from build123d import *

# Parameters (mm, degrees)
F0_R     = 4.5
F0_R_2   = 2.95
F1_DEPTH = 10
F0_R_3   = 15.5
F2_DEPTH = 10
F3_DEPTH = 15


with BuildPart() as f1:
    # F0 (on Top) → F1 (new body)
    with BuildSketch(Plane.XY):
        Circle(F0_R)
        Circle(F0_R_2, mode=Mode.SUBTRACT)
    extrude(amount=F1_DEPTH)

    # F0 (on Top) → F2 (join)
    with BuildSketch(Plane.XY):
        Circle(F0_R_3)
        Circle(F0_R, mode=Mode.SUBTRACT)
    extrude(amount=-F2_DEPTH)

    # F3 (add): a face of the model
    f3_faces = [f1.faces().sort_by_distance(p)[0] for p in [
        (-4.3727207794, 0, 0),
    ]]
    extrude(f3_faces, amount=F3_DEPTH)


solid = f1.part
The listing builds one solid part. Answer for the finished solid, in the listing's coordinates (mm). A direction names the side the tool comes from. Coordinates: 2 decimals unless noted, no trailing zeros. Order: outer loops, then holes, each group sorted by start corner. A loop starts at its lowest first (then second) coordinate and runs counter-clockwise, first axis right, second up. Notation, with made-up numbers: (82.5, 77.5) -> (98.5, 77.5) arc R21 cw to (98.5, 99.5) -> close; hole circle Ø9 at (21, 73). An arc over 180 degrees is marked (long way). Answer in a Markdown table with one row per item. Add a question column.
Item 1: Find section D-D (x = 8). Write down the section's boundary in (y, z), then the cut area to 3 significant figures.
Item 2: Which of the six approach directions +Z, -Z, +X, -X, +Y, -Y give full straight-line access (tool end or side, diameter ignored) to faces 1 (the face through (1, -3, -15)), 2 (the face through (-4, -3, -10)), 3 (the face through (-0.59, 4.46, 4.93))?
Item 3: Find section C-C (z = -1.5). Write down the section's boundary in (x, y), then the cut area to 3 significant figures.
Item 4: Each of these flat-tipped pins is pushed along its axis until it touches: P1, Ø10, axis at x = 10, y = -5, coming from the -Z side; P2, Ø5.5, axis at x = 0, y = 0, coming from the +Z side; P3, Ø5, axis at y = -4.5, z = -1, coming from the +X side; P4, Ø10, axis at y = 11, z = -6, coming from the +X side. Where does it stop, or does it pass through?
Item 5: Find the intervals of material crossed by L1, parallel to Y at x = 0, z = -10.75; L2, parallel to Y at x = 0, z = -5.75; L3, parallel to Z at x = -10, y = -1, in increasing order. Write a range as from..to.
Item 6: Find section A-A (x = 0). Write down the section's boundary in (y, z), then the cut area to 4 significant figures.
Result set:
| question | item | result |
|---|---|---|
| 1 | outline | (-13.28, -10) -> (13.28, -10) -> (13.28, 0) -> (-13.28, 0) -> close |
| 1 | area | 266 mm² |
| 2 | face 1 | -Z, +X, -X, +Y, -Y |
| 2 | face 2 | -Z |
| 2 | face 3 | +Z |
| 3 | outline | circle Ø31 at (0, 0); hole circle Ø5.9 at (0, 0) |
| 3 | area | 727 mm² |
| 4 | P1 | stops at z = -10 |
| 4 | P2 | passes through |
| 4 | P3 | stops at x = 15.37 |
| 4 | P4 | stops at x = 14.29 |
| 5 | L1 | y = -4.5..-2.95, 2.95..4.5 |
| 5 | L2 | y = -15.5..-2.95, 2.95..15.5 |
| 5 | L3 | z = -10..0 |
| 6 | outline | (-15.5, -10) -> (-4.5, -10) -> (-4.5, -15) -> (-2.95, -15) -> (-2.95, 10) -> (-4.5, 10) -> (-4.5, 0) -> (-15.5, 0) -> close; (2.95, -15) -> (4.5, -15) -> (4.5, -10) -> (15.5, -10) -> (15.5, 0) -> (4.5, 0) -> (4.5, 10) -> (2.95, 10) -> close |
| 6 | area | 297.5 mm² |
